Source: CAD feature listing. Evaluate the final solid. Frame: model axes, mm. Round coordinates to 2 decimals unless told otherwise and drop trailing zeros. Write each loop counter-clockwise with the first axis right and the second up, starting at its lowest first coordinate (ties: lowest second). Pieces come first, ordered by that corner, then holes.
from build123d import *

# Parameters (mm, degrees)
SKETCH1_W           = 120
SKETCH1_H           = 120
SKETCH1_R           = 11.05
SKETCH1_R_2         = 1.5
SKETCH1_R_3         = 2.5
SKETCH1_R_4         = 2.85
BOSS_EXTRUDE1_DEPTH = 8
SKETCH3_W           = 169.939825448
SKETCH3_H           = 19.036974982
SKETCH3_W_2         = 188.744642198
SKETCH3_H_2         = 29.251937167
CUT_EXTRUDE1_DEPTH  = 10
SKETCH4_R           = 4.25
CUT_EXTRUDE2_DEPTH  = 6
SKETCH5_R           = 2.5
CUT_EXTRUDE3_DEPTH  = 131.245921241


with BuildPart() as part:
    # Sketch1 → Boss-Extrude1 (new body)
    with BuildSketch(Plane.XY):
        with Locations((-60, 0)):
            Rectangle(SKETCH1_W, SKETCH1_H)
        with Locations((-98.5, 0)):
            Circle(SKETCH1_R, mode=Mode.SUBTRACT)
        with Locations((-83, 15.5)):
            Circle(SKETCH1_R_2, mode=Mode.SUBTRACT)
        with Locations((-114, 15.5)):
            Circle(SKETCH1_R_2, mode=Mode.SUBTRACT)
        with Locations((-114, -15.5)):
            Circle(SKETCH1_R_2, mode=Mode.SUBTRACT)
        with Locations((-83, -15.5)):
            Circle(SKETCH1_R_2, mode=Mode.SUBTRACT)
        with Locations((-61.5, 37.5)):
            Circle(SKETCH1_R_3, mode=Mode.SUBTRACT)
        with Locations((-28.5, 37.5)):
            Circle(SKETCH1_R_3, mode=Mode.SUBTRACT)
        with Locations((-61.5, 11.5)):
            Circle(SKETCH1_R_3, mode=Mode.SUBTRACT)
        with Locations((-28.5, 11.5)):
            Circle(SKETCH1_R_3, mode=Mode.SUBTRACT)
        with Locations((-61.5, -11.5)):
            Circle(SKETCH1_R_3, mode=Mode.SUBTRACT)
        with Locations((-28.5, -11.5)):
            Circle(SKETCH1_R_3, mode=Mode.SUBTRACT)
        with Locations((-28.5, -37.5)):
            Circle(SKETCH1_R_3, mode=Mode.SUBTRACT)
        with Locations((-61.5, -37.5)):
            Circle(SKETCH1_R_3, mode=Mode.SUBTRACT)
        with Locations((-15, 45.1)):
            Circle(SKETCH1_R_4, mode=Mode.SUBTRACT)
        with Locations((-15, 13)):
            Circle(SKETCH1_R_4, mode=Mode.SUBTRACT)
        with Locations((-15, -13)):
            Circle(SKETCH1_R_4, mode=Mode.SUBTRACT)
        with Locations((-15, -45.1)):
            Circle(SKETCH1_R_4, mode=Mode.SUBTRACT)
    extrude(amount=BOSS_EXTRUDE1_DEPTH)

    # Sketch3 → Cut-Extrude1 (cut)
    with BuildSketch(Plane.XY.offset(8)):
        with Locations((-54.971186983, 59.518487491)):
            Rectangle(SKETCH3_W, SKETCH3_H)
        with Locations((-45.568778608, -64.625968583)):
            Rectangle(SKETCH3_W_2, SKETCH3_H_2)
    extrude(amount=-CUT_EXTRUDE1_DEPTH, mode=Mode.SUBTRACT)

    # Sketch4 → Cut-Extrude2 (cut)
    with BuildSketch(Plane.XY.offset(8)):
        with Locations((-61.5, 37.5)):
            Circle(SKETCH4_R)
        with Locations((-28.5, 37.5)):
            Circle(SKETCH4_R)
        with Locations((-61.5, 11.5)):
            Circle(SKETCH4_R)
        with Locations((-28.5, 11.5)):
            Circle(SKETCH4_R)
        with Locations((-61.5, -11.5)):
            Circle(SKETCH4_R)
        with Locations((-28.5, -11.5)):
            Circle(SKETCH4_R)
        with Locations((-61.5, -37.5)):
            Circle(SKETCH4_R)
        with Locations((-28.5, -37.5)):
            Circle(SKETCH4_R)
    extrude(amount=-CUT_EXTRUDE2_DEPTH, mode=Mode.SUBTRACT)

    # Sketch5 → Cut-Extrude3 (cut, through all)
    with BuildSketch(Plane.XY.offset(8)):
        with Locations((-15, 0)):
            Circle(SKETCH5_R)
        with Locations((-59, 0)):
            Circle(SKETCH5_R)
    extrude(amount=-CUT_EXTRUDE3_DEPTH, mode=Mode.SUBTRACT)


solid = part.part
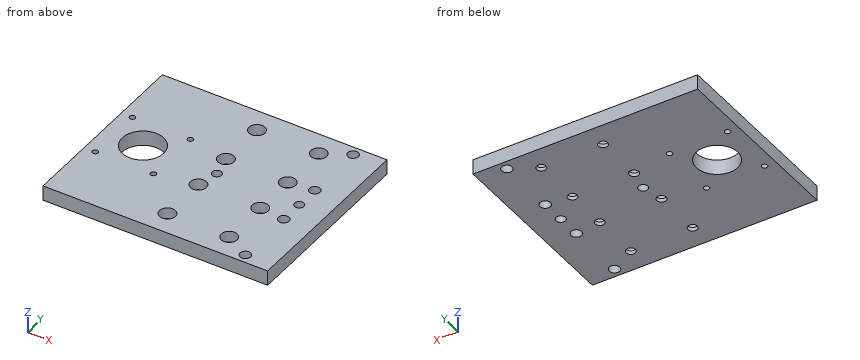
1) Material intervals for line 1 (Y direction, x = -15, z = 5.5); line 2 (Y direction, x = -28.5, z = 3.35); line 3 (X direction, y = -37.5, z = 1.2), sorted ascending.
Taken from the geometry:
line 1: y = -50 to -47.95, -42.25 to -15.85, -10.15 to -2.5, 2.5 to 10.15, 15.85 to 42.25, 47.95 to 50
line 2: y = -50 to -41.75, -33.25 to -15.75, -7.25 to 7.25, 15.75 to 33.25, 41.75 to 50
line 3: x = -120 to -64, -59 to -31, -26 to 0
2) Section query B-B on x = -114. Return the cut outline in (y, z), then the cut area to 3 significant figures.
Taken from the geometry:
outline: (-50, 0) - (-17, 0) - (-17, 8) - (-50, 8) - close; (-14, 0) - (14, 0) - (14, 8) - (-14, 8) - close; (17, 0) - (50, 0) - (50, 8) - (17, 8) - close
area: 752 mm2
3) Section query A-A on y = -37.5. Return the cut outline in (x, z), then the cut area to 3 significant figures.
Taken from the geometry:
outline: (-120, 0) - (-64, 0) - (-64, 2) - (-65.75, 2) - (-65.75, 8) - (-120, 8) - close; (-59, 0) - (-31, 0) - (-31, 2) - (-32.75, 2) - (-32.75, 8) - (-57.25, 8) - (-57.25, 2) - (-59, 2) - close; (-26, 0) - (0, 0) - (0, 8) - (-24.25, 8) - (-24.25, 2) - (-26, 2) - close
area: 838 mm2
4) Contact query for flat-ended pins moving along their axis: P1, Ø7.5, axis at x = -61.5, y = -37.5, coming from the +Z side; P2, Ø2, axis at x = -103.5, y = -27.5, coming from the -Z side; P3, Ø4, axis at x = -15, y = 0, coming from the -Z side. Output: stop coordinate, or through.
Taken from the geometry:
P1: stops at z = 2
P2: stops at z = 0
P3: passes through
5) Section query D-D on y = 45.1. Return the cut outline in (x, z), then the cut area to 3 significant figures.
Taken from the geometry:
outline: (-120, 0) - (-17.85, 0) - (-17.85, 8) - (-120, 8) - close; (-12.15, 0) - (0, 0) - (0, 8) - (-12.15, 8) - close
area: 914 mm2
6) Section query C-C on z = 3.5. State how many separate pieces and enclosed holes the cut face has, then the cut area to 3 significant figures.
Taken from the geometry:
separate pieces: 1
enclosed holes: 19
area: 11,000 mm2
